Autodesk Inventor part; units mm, degrees
ref_plane "YZ Plane" through (0, 0, 0) normal (1, 0, 0) x (0, 1, 0)
ref_plane "XZ Plane" through (0, 0, 0) normal (0, 1, 0) x (-1, 0, 0)
ref_plane "XY Plane" through (0, 0, 0) normal (0, 0, 1) x (1, 0, 0)
sketch "Sketch1" plane through (0, 0, 0) normal (0, 1, 0) x (-1, 0, 0)
  line L0 (198.4375, 333.375) -> (198.4375, -333.375)
  line L1 (198.4375, -333.375) -> (-198.4375, -333.375)
  line L2 (-198.4375, -333.375) -> (-198.4375, 333.375)
  line L3 (-198.4375, 333.375) -> (198.4375, 333.375)
  line L4 (198.4375, 333.375) -> (-198.4375, -333.375) construction
  line L5 (198.4375, -333.375) -> (-198.4375, 333.375) construction
  point P0 (0, 0)
  dimension "d0" = 666.75
  dimension "d1" = 396.875
extrude "Extrusion1" add sketch "Sketch1" along normal blind 6.35
sketch "Sketch2" plane through (0, 6.35, 0) normal (0, 1, 0) x (1, 0, 0)
  line L0 (179.3875, -155.575) -> (103.1875, -155.575)
  line L1 (103.1875, -155.575) -> (103.1875, -130.175)
  line L2 (103.1875, -130.175) -> (179.3875, -130.175)
  line L3 (179.3875, -130.175) -> (179.3875, -155.575)
  line L4 (198.4375, -333.375) -> (198.4375, 333.375)
  line L5 (-179.3875, -155.575) -> (-103.1875, -155.575)
  line L6 (-103.1875, -155.575) -> (-103.1875, -130.175)
  line L7 (-103.1875, -130.175) -> (-179.3875, -130.175)
  line L8 (-179.3875, -130.175) -> (-179.3875, -155.575)
  line L9 (-198.4375, 333.375) -> (-198.4375, -333.375)
  line L10 (198.4375, -333.375) -> (-198.4375, -333.375)
  point P0 (0, 0)
  dimension "d4" = 76.2
  dimension "d5" = 25.4
  dimension "d6" = 19.05
  dimension "d7" = 76.2
  dimension "d8" = 25.4
  dimension "d9" = 19.05
  dimension "d10" = 177.8
  dimension "d11" = 177.8
extrude "Extrusion2" add sketch "Sketch2" along normal blind 76.2
sketch "Sketch3" plane through (-179.3875, 6.35, 155.575) normal (0, 0, 1) x (1, 0, 0)
  circle A0 centre (38.1, 38.1) radius 19.05
  circle A1 centre (228.6, 38.1) radius 19.05
  point P0 (179.3875, -6.35)
  dimension "d14" = 38.1
  dimension "d15" = 38.1
extrude "Extrusion3" cut sketch "Sketch3" against normal blind 76.2
sketch "Sketch4" plane through (-179.3875, 6.35, 155.575) normal (0, 0, 1) x (1, 0, 0)
  circle A0 centre (38.1, 38.1) radius 19.05
  circle A1 centre (38.1, 38.1) radius 19.05
  circle A2 centre (320.675, 38.1) radius 19.05
  point P0 (179.3875, -6.35)
  dimension "d44" = 38.1
extrude "Extrusion4" add sketch "Sketch4" along normal blind 88.9 and the other way blind 88.9
sketch "Sketch5" plane through (49.2125, 44.45, 66.675) normal (0, 0, -1) x (-1, 0, 0)
  circle A0 centre (190.5, 0) radius 19.05
  circle A1 centre (190.5, 0) radius 38.1
  circle A2 centre (-92.075, 0) radius 19.05
  circle A3 centre (-92.075, 0) radius 38.1
  point P0 (49.2125, -44.45)
  dimension "d23" = 76.2
extrude "Extrusion5" add sketch "Sketch5" along normal blind 508 contours A0 | A1 | A2 | A3
sketch "Sketch6" plane through (-141.2875, 44.45, 244.475) normal (0, 0, 1) x (1, 0, 0)
  line L0 (-22.225, -22.225) -> (22.225, -22.225)
  line L1 (22.225, -22.225) -> (22.225, 22.225)
  line L2 (22.225, 22.225) -> (-22.225, 22.225)
  line L3 (-22.225, 22.225) -> (-22.225, -22.225)
  line L4 (-22.225, -22.225) -> (22.225, 22.225) construction
  line L5 (22.225, -22.225) -> (-22.225, 22.225) construction
  line L6 (304.8, -22.225) -> (260.35, -22.225)
  line L7 (260.35, -22.225) -> (260.35, 22.225)
  line L8 (260.35, 22.225) -> (304.8, 22.225)
  line L9 (304.8, 22.225) -> (304.8, -22.225)
  line L10 (304.8, -22.225) -> (260.35, 22.225) construction
  line L11 (260.35, -22.225) -> (304.8, 22.225) construction
  line L12 (-38.1, -38.1) -> (-38.1, 38.1)
  line L13 (-38.1, 38.1) -> (38.1, 38.1)
  point P0 (141.2875, -44.45)
  point P1 (0, 0)
  point P2 (282.575, 0)
  dimension "d26" = 44.45
  dimension "d27" = 44.45
  dimension "d28" = 44.45
  dimension "d29" = 44.45
  dimension "d30" = 282.575
  dimension "d31" = 38.1
  dimension "d32" = 38.1
extrude "Extrusion6" add sketch "Sketch6" along normal blind 38.1
sketch "Sketch7" plane through (119.0625, 22.225, 244.475) normal (-1, 0, 0) x (0, 0, 1)
  circle A0 centre (19.05, 19.05) radius 19.05
  line L0 (0, 0) -> (0, 44.45)
  line L1 (0, 0) -> (38.1, 0)
  point P0 (-244.475, -22.225)
  dimension "d35" = 38.1
  dimension "d36" = 19.05
  dimension "d37" = 19.05
extrude "Extrusion7" add sketch "Sketch7" along normal blind 238.125 contours A0
sketch "Sketch9" plane through (-141.2875, 44.45, -441.325) normal (0, 0, -1) x (-1, 0, 0)
  circle A0 centre (0, 0) radius 36.5125
  point P0 (-141.2875, -44.45)
  dimension "d45" = 73.025
extrude "Extrusion9" cut sketch "Sketch9" against normal blind 501.65
properties part number "Cannon Barrel"
For this review, take the finished solid that the model builds, in its own axes (mm). A direction names the side the tool comes from. Coordinates: 2 decimals unless noted, no trailing zeros. Order: outer loops, then holes, each group sorted by start corner. A loop starts at its lowest first (then second) coordinate and runs counter-clockwise, first axis right, second up. Notation, with made-up numbers: (61.25, 7.5) -> (115.25, 7.5) arc R32 cw to (115.25, 37.5) -> close; hole circle Ø7 at (65.25, 89.5). An arc over 180 degrees is marked (long way). Answer as CSV lines item,"result".
Q1. Wall thickness on line 1 along X through (y, z) = (47, -61.5); line 2 along X through (y, z) = (45, -407); line 3 along Z through (x, y) = (126, 32) (3 decimals): over which ranges is each line inside the solid? List them lowest first. Write a range as [from, to].
Model answer:
line 1,"x = [-179.3, -177.71], [-104.86, -103.27], [103.27, 179.3]"
line 2,"x = [-179.38, -177.8], [-104.78, -103.19], [103.19, 179.38]"
line 3,"z = [-441.325, 66.675], [130.175, 155.575], [244.475, 282.575]"
Q2. Draft analysis for pull direction Z (two halves, no side actions). For faces 1 (the face through (-141, 45, 60.325)), 2 (the face through (3, 0, 5)), 3 (the face through (119.062, 26, 249)), state which applies: released by +Z, released by -Z, zero draft, split by the parting line, or undercut.
Model answer:
face 1,"released by -Z"
face 2,"zero draft"
face 3,"undercut"
Q3. We need section B-B (z = 18.5). Count the separate pieces of the cut face and the enclosed holes in it, plus the area to 3 significant figures.
Model answer:
separate pieces,"3"
enclosed holes,"1"
area,"7,450 mm2"
Q4. For faces 4 (the face through (1.667, 48.571, 281.122)), 5 (the face through (-179.388, 44, 143)), 6 (the face through (-163.512, 45, 263)), 7 (the face through (163.512, 45, 263)), 8 (the face through (-119.062, 26, 278)), list the 3-axis set-ups (+Z, -Z, +X, -X, +Y, -Y) from which the entire face can be reached by the end or side of a thin tool; tool diameter is ignored.
Model answer:
face 4,"none"
face 5,"+Z, -Z, -X, +Y"
face 6,"+Z, -X, +Y"
face 7,"+Z, +X, +Y"
face 8,"+Z"
Q5. We need section C-C (z = 142.5). State the section outline as (x, y) points.
Model answer:
outline,"(-198.44, 0) -> (198.44, 0) -> (198.44, 6.35) -> (179.39, 6.35) -> (179.39, 82.55) -> (103.19, 82.55) -> (103.19, 6.35) -> (-103.19, 6.35) -> (-103.19, 82.55) -> (-179.39, 82.55) -> (-179.39, 6.35) -> (-198.44, 6.35) -> close"
Q6. We need section A-A (x = 1). State the section outline as (y, z) points (3 decimals), plus the area to 3 significant figures.
Model answer:
outline,"(0, -333.375) -> (6.35, -333.375) -> (6.35, 333.375) -> (0, 333.375) -> close; circle Ø38.1 at (41.275, 263.525)"
area,"5,370 mm2"
Q7. Clearance check with flat-ended pins moving along their axes: pin 1 Ø10 at (x, y) = (-94.5, 69) entering from -Z; pin 2 Ø1 at (y, z) = (10.5, -172.5) entering from +X; pin 3 Ø1 at (y, z) = (28.5, -11.5) entering from +X; pin 4 Ø20.5 at (y, z) = (57.5, 255.5) entering from -X. State where each tip first meets the part, or that it passes through.
Model answer:
pin 1,"passes through"
pin 2,"stops at x = 159.53"
pin 3,"stops at x = 176.11"
pin 4,"stops at x = -163.51"
